from build123d import *

# Parameters (mm, degrees)
SKETCH_1_R          = 1.5
EXTRUDE_1_DEPTH     = 8
SKETCH_2_W          = 12
SKETCH_2_H          = 3
CUT_EXTRUDE_1_DEPTH = 48.201694885
SKETCH_3_R          = 0.9
CUT_EXTRUDE_2_DEPTH = 6
SKETCH_4_W          = 20.5
SKETCH_4_H          = 7.5
CUT_EXTRUDE_3_DEPTH = 1.5
FILLET_2_R          = 3
FILLET_3_R          = 3


with BuildPart() as part:
    # 草图1 → 凸台-拉伸1 (new body)
    with BuildSketch(Plane(origin=(0, 0, 0), x_dir=(1, 0, 0), z_dir=(0, 1, 0))):
        Polygon((0, 0), (42, 0), (42, 3), (30, 8), (30, 20), (0, 20), align=None)
        with Locations(Location((25, 16, 0), (0, 0, 270))):
            Circle(SKETCH_1_R, mode=Mode.SUBTRACT)
        with Locations(Location((5, 16, 0), (0, 0, 270))):
            Circle(SKETCH_1_R, mode=Mode.SUBTRACT)
    extrude(amount=EXTRUDE_1_DEPTH)

    # 草图2 → 切除-拉伸1 (cut, through all)
    with BuildSketch(Plane.ZY):
        Polygon((-20, 6), (-10, 6), (-8, 8), (-20, 8), align=None)
        with Locations((-14, 1.5)):
            Rectangle(SKETCH_2_W, SKETCH_2_H)
    extrude(amount=-CUT_EXTRUDE_1_DEPTH, mode=Mode.SUBTRACT)

    # 草图3 → 切除-拉伸2 (cut)
    with BuildSketch(Plane.XY):
        with Locations((26.5, 3.5)):
            Circle(SKETCH_3_R)
        with Locations((36, 3.5)):
            Circle(SKETCH_3_R)
    extrude(amount=-CUT_EXTRUDE_2_DEPTH, mode=Mode.SUBTRACT)

    # 草图4 → 切除-拉伸3 (cut)
    with BuildSketch(Plane.XY):
        with Locations((31.25, 3.75)):
            Rectangle(SKETCH_4_W, SKETCH_4_H)
    extrude(amount=-CUT_EXTRUDE_3_DEPTH, mode=Mode.SUBTRACT)

    # 圆角2
    fillet_2_edges = [part.edges().sort_by_distance(p)[0] for p in [
        (0, 4.5, -20),
        (30, 4.5, -20),
        (42, 4, -3),
        (30, 5.5, -8),
    ]]
    fillet(fillet_2_edges, radius=FILLET_2_R)

    # 圆角3
    fillet_3_edges = [part.edges().sort_by_distance(p)[0] for p in [
        (30, 1.5, -8),
    ]]
    fillet(fillet_3_edges, radius=FILLET_3_R)


solid = part.part
For this review, take the finished solid that the model builds, in its own axes (mm). A direction names the side the tool comes from. Round coordinates to 2 decimals unless told otherwise and drop trailing zeros. Order: outer loops, then holes, each group sorted by start corner. A loop starts at its lowest first (then second) coordinate and runs counter-clockwise, first axis right, second up. Notation, with made-up numbers: (61, 4) -> (94, 4) arc R20 cw to (94, 24) -> close; hole circle Ø3 at (13.25, -9). An arc over 180 degrees is marked (long way). Put each result on its own line as item: value.
Q1. Add section C-C on y = 5.25. Write out the cut boundary in (x, z), plus the area to 3 significant figures.
Check result:
outline: (0, -17) arc R3 ccw to (3, -20) -> (27, -20) arc R3 ccw to (30, -17) -> (30, -10) arc R3 cw to (31.85, -7.23) -> (40.15, -3.77) arc R3 ccw to (42, -1) -> (42, 0) -> (41.5, 0) -> (41.5, -1.5) -> (21, -1.5) -> (21, 0) -> (0, 0) -> close; hole circle Ø3 at (5, -16); hole circle Ø3 at (25, -16)
area: 617 mm2
Q2. Machinability: for faces 4 (the cylindrical face through (26.915, 2.702, -3.718)), 5 (the flat face through (31, 4, -1.5)), 6 (the cylindrical face through (30, 1.52, -7.94)), which of the approach directions +Z, -Z, +X, -X, +Y, -Y give a long, thin tool a straight path to every point of the face, cutting with its end or side? Answer none if there is none.
Check result:
face 4: +Z
face 5: +Z, -Y
face 6: -Z, +X, -Y
Q3. Insertion check: pin 1 Ø1 at (x, y) = (37, 6.5) entering from -Z; pin 2 Ø2 at (x, y) = (26.5, 5.5) entering from +Z; pin 3 Ø1.5 at (x, z) = (26, -14) entering from -Y. Each pin has a flat end and moves straight along its axis. Give the tip position at first contact, or say it passes through.
Check result:
pin 1: z = -5.29
pin 2: z = -1.5
pin 3: y = 3
Q4. For probe 1 along X at (y, z) = (4.5, -16); probe 2 along X at (y, z) = (4.25, -15.5); probe 3 along Z at (x, y) = (5, 4.55), list the stretches that pass through material, from the lowest coordinate up. Write a range as [from, to].
Check result:
probe 1: [0, 3.5], [6.5, 23.5], [26.5, 30]
probe 2: [0, 3.59], [6.41, 23.59], [26.41, 30]
probe 3: [-20, -17.5], [-14.5, 0]
Q5. Add section D-D on y = 3.5. Write out the cut boundary in (x, z) (3 decimals).
Check result:
outline: (0, -17) arc R3 ccw to (3, -20) -> (27, -20) arc R3 ccw to (30, -17) -> (30, -10) arc R3 cw to (31.846, -7.231) -> (35.1, -5.875) -> (35.1, -1.5) -> (27.4, -1.5) -> (27.4, -6) -> (25.6, -6) -> (25.6, -1.5) -> (21, -1.5) -> (21, 0) -> (0, 0) -> close; (36.9, -5.125) -> (40.154, -3.769) arc R3 ccw to (42, -1) -> (42, 0) -> (41.5, 0) -> (41.5, -1.5) -> (36.9, -1.5) -> close; hole circle Ø3 at (5, -16); hole circle Ø3 at (25, -16)
Q6. Mouldability with a two-part tool opening along X and no side actions: class faces 1 (the flat face through (16, 0, -4)), 2 (the cylindrical face through (30.518, 5.535, -8.315)), 3 (the cylindrical face through (35.1, 3.5, -3.7)) as pulls with the +X half, pulls with the -X half, needs draft (parallel to the pull), parting line crosses it, or undercut.
Check result:
face 1: needs draft
face 2: pulls with the +X half
face 3: undercut
Q7. Add section A-A on x = 36. Write out the cut boundary in (y, z), plus the area to 4 significant figures.
Check result:
outline: (0, -5.5) -> (2.6, -5.5) -> (2.6, -1.5) -> (0, -1.5) -> close; (4.4, -5.5) -> (8, -5.5) -> (8, 0) -> (7.5, 0) -> (7.5, -1.5) -> (4.4, -1.5) -> close
area: 25.55 mm2
Q8. Add section B-B on z = -16. Write out the cut boundary in (x, y).
Check result:
outline: (0, 3) -> (3.5, 3) -> (3.5, 6) -> (0, 6) -> close; (6.5, 3) -> (23.5, 3) -> (23.5, 6) -> (6.5, 6) -> close; (26.5, 3) -> (30, 3) -> (30, 6) -> (26.5, 6) -> close
